from build123d import *

# Parameters (mm, degrees)
BOSS_EXTRUDE1_DEPTH = 52
FILLET1_R           = 25
CUT_EXTRUDE1_DEPTH  = 52
FILLET2_R           = 10
SKETCH3_R           = 12.5
CUT_EXTRUDE2_DEPTH  = 52
SKETCH5_W           = 63.955413662
SKETCH5_H           = 6.318805718
BOSS_EXTRUDE2_DEPTH = 52
SKETCH6_R           = 14.796953782
CUT_EXTRUDE5_DEPTH  = 12


with BuildPart() as part:
    # Sketch1 → Boss-Extrude1 (new body)
    with BuildSketch(Plane(origin=(0, 0, 0), x_dir=(1, 0, 0), z_dir=(0, 1, 0))):
        Polygon((0, 0), (-54.007699651, 24.646064638), (-58.048980527, 15.790278249), (0, -10.699998794), (55, 8.034068022), (55, 18.734066816), align=None)
    extrude(amount=-BOSS_EXTRUDE1_DEPTH)

    # Fillet1
    fillet1_edges = [part.edges().sort_by_distance(p)[0] for p in [
        (55, -52, -13.384067419),
        (55, 0, -13.384067419),
    ]]
    fillet(fillet1_edges, radius=FILLET1_R)

    # Sketch2 → Cut-Extrude1 (cut)
    with BuildSketch(Plane(origin=(3.265731793, 0, 9.587627201), x_dir=(0.9465939078280105, 0, -0.32242824575848833), z_dir=(0.32242824575848833, 0, 0.9465939078280106))):
        with BuildLine():
            Line((54.653075389, -38.5), (23.959854488, -38.5))
            ThreePointArc((23.959854488, -38.5), (11.459854488, -26), (23.959854488, -13.5))
            Line((23.959854488, -13.5), (54.653075389, -13.5))
            ThreePointArc((54.653075389, -13.5), (67.153075389, -26), (54.653075389, -38.5))
        make_face()
    extrude(amount=-CUT_EXTRUDE1_DEPTH, mode=Mode.SUBTRACT)

    # Fillet2
    fillet2_edges = [part.edges().sort_by_distance(p)[0] for p in [
        (-56.028340089, 0, -20.218171443),
    ]]
    fillet(fillet2_edges, radius=FILLET2_R)

    # Sketch3 → Cut-Extrude2 (cut)
    with BuildSketch(Plane(origin=(-4.041280876, 0, 8.855786388), x_dir=(0.9097492407271736, 0, 0.4151581855104526), z_dir=(-0.4151581855104526, 0, 0.9097492407271736))):
        with Locations((-30.557807916, -26)):
            Circle(SKETCH3_R)
    extrude(amount=-CUT_EXTRUDE2_DEPTH, mode=Mode.SUBTRACT)

    # Sketch5 → Boss-Extrude2 (add)
    with BuildSketch(Plane(origin=(-4.041280876, 0, 8.855786388), x_dir=(0.9097492407271736, 0, 0.4151581855104526), z_dir=(-0.4151581855104526, 0, 0.9097492407271736))):
        with Locations((-27.387772395, -48.840597141)):
            Rectangle(SKETCH5_W, SKETCH5_H)
    extrude(amount=BOSS_EXTRUDE2_DEPTH)

    # Sketch6 → Cut-Extrude5 (cut)
    with BuildSketch(Plane(origin=(0, -45.681194282, 0), x_dir=(1, 0, 0), z_dir=(0, 1, 0))):
        with Locations(Location((-41.275083904, -23.507254491, 0), (0, 0, 270))):
            Circle(SKETCH6_R)
        with BuildLine():
            add(Edge.make_bspline(
                [(-58.048980527, 15.790278249), (-55.831409205, 12.43111817), (-55.468462462, -1.484994571), (-66.211863789, -17.980786489), (-64.125030252, -34.334258251), (-56.260496604, -41.858023354), (-51.107014647, -44.526823974), (-50.545511664, -44.792489014)],
                knots=[0, 0, 0, 0, 0.058811155, 0.20931912, 0.241844454, 0.351539163, 0.365251001, 0.365251001, 0.365251001, 0.365251001], degree=3))
            Line((-58.048980527, 15.790278249), (-79.637206174, -31.516682269))
            Line((-79.637206174, -31.516682269), (-50.545511664, -44.792489014))
        make_face()
        with BuildLine():
            add(Edge.make_bspline(
                [(-49.907067766, -45.08383876), (-49.177932221, -45.404712271), (-41.127943342, -48.502484641), (-33.005537612, -48.370799962), (-20.855856008, -36.685330942), (-16.080658073, -18.863651279), (-4.727836106, -10.381149917), (0, -10.699998794)],
                knots=[0.370486493, 0.370486493, 0.370486493, 0.370486493, 0.388554906, 0.574986146, 0.630925752, 0.892011359, 1, 1, 1, 1], degree=3))
            Line((-49.907067766, -45.08383876), (-21.453817154, -58.068295759))
            Line((-21.453817154, -58.068295759), (0.134408493, -10.761335241))
            Line((0.134408493, -10.761335241), (0, -10.699998794))
        make_face()
    extrude(amount=-CUT_EXTRUDE5_DEPTH, mode=Mode.SUBTRACT)


solid = part.part
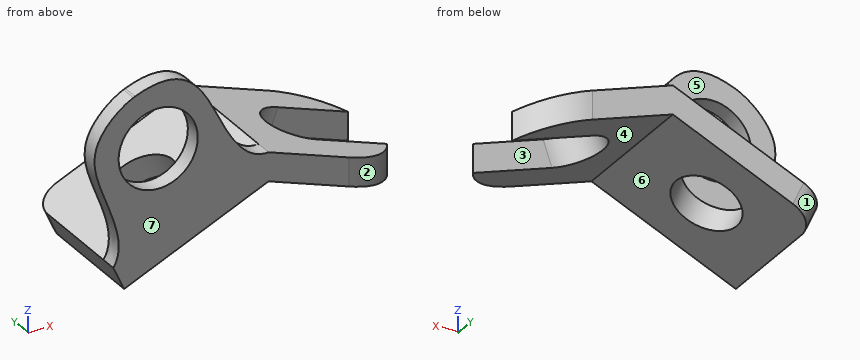
Geometry check sheet. Reference: the model listing, model coordinates, mm. Face numbers are marked on the shaded views. A direction names the side the tool comes from. Give positions to 0.01 mm unless a question says otherwise; leave off trailing zeros. Order: outer loops, then holes, each group sorted by start corner. A loop starts at its lowest first (then second) coordinate and runs counter-clockwise, first axis right, second up. Notation, with made-up numbers: (-26.5, -20.75) - (23.5, -20.75) arc R25 cw to (23.5, -7.75) - close; hole circle Ø5 at (10.25, 65). An arc over 180 degrees is marked (long way). Answer as a JSON object with one key per item and string values.
(1) Draft check along Y on the marked faces 1, 2, 3 and 4. Enter one of: released by +Y, released by -Y, zero draft, split by the parting line, or undercut.
Report:
{"face 1": "released by +Y", "face 2": "released by -Y", "face 3": "undercut", "face 4": "zero draft"}
(2) Material ranges on line 1 (X direction, y = -49, z = 15); line 2 (Z direction, x = 11, y = -47.5); line 3 (Z direction, x = -1, y = -5.5), recorded low to high.
Report:
{"line 1": "-62.95 to -53.38, -29.17 to -9.89", "line 2": "-3.75 to 6.95", "line 3": "-0.46 to 10.24"}
(3) Cross-section at A-A (y = -23). Record the cut outline in (x, z).
Report:
{"outline": "(-58.05, -15.79) - (-54.01, -24.65) - (-38.84, -17.72) - (-42.88, -8.87) - close; (-20.8, 1.21) - (-16.76, -7.65) - (0, 0) - (11.19, -3.81) - (14.46, 5.77) - (0, 10.7) - close"}
(4) Cross-section at B-B (y = -15). Record the cut outline in (x, z), then the cut area to 3 significant figures.
Report:
{"outline": "(-58.05, -15.79) - (-54.01, -24.65) - (-33.2, -15.15) - (-37.24, -6.3) - close; (-26.44, -1.37) - (-22.4, -10.22) - (0, 0) - (17.06, -5.81) - (20.33, 3.78) - (0, 10.7) - close", "area": "684 mm^2"}
(5) Tool access check on the marked faces 5, 6 and 7. Record the directions out of +Z, -Z, +X, -X, +Y, -Y that give a thin tool (end or side, any length) a straight path to the whole face; none if there is none.
Report:
{"face 5": "+Z, -X, +Y", "face 6": "-Z, +Y, -Y", "face 7": "+Z, -Z, +X, -X, -Y"}
(6) Cross-section at C-C (y = -43). Record the cut outline in (x, z), then the cut area to 3 significant figures.
Report:
{"outline": "(-58.05, -15.79) - (-54.01, -24.65) - (0, 0) - (49.21, -16.76) - (49.21, -6.06) - (0, 10.7) - close", "area": "1,130 mm^2"}
(7) Depth check by flat-ended pin: pin 1 Ø8 at (y, z) = (-24, 4) entering from +X; pin 2 Ø10 at (y, z) = (-34, -5) entering from +X; pin 3 Ø9.5 at (x, z) = (41.5, -4) entering from -Y. Enter the tip coordinate at first touch or a pass-through.
Report:
{"pin 1": "x = 15.43", "pin 2": "x = 52.2", "pin 3": "y = -51.07"}
